from build123d import *

# Parameters (mm, degrees)
ESQUISSE1_W        = 256
ESQUISSE1_H        = 350
BOSS_EXTRU_1_DEPTH = 10
ESQUISSE2_W        = 256
ESQUISSE2_H        = 350
ESQUISSE2_W_2      = 236
ESQUISSE2_H_2      = 330
BOSS_EXTRU_2_DEPTH = 70
ESQUISSE3_W        = 10
ESQUISSE3_H        = 330
BOSS_EXTRU_3_DEPTH = 70


with BuildPart() as part:
    # Esquisse1 → Boss.-Extru.1 (new body)
    with BuildSketch(Plane.XY):
        with Locations((128, 175)):
            Rectangle(ESQUISSE1_W, ESQUISSE1_H)
    extrude(amount=BOSS_EXTRU_1_DEPTH)

    # Esquisse2 → Boss.-Extru.2 (add)
    with BuildSketch(Plane.XY.offset(10)):
        with Locations((128, 175)):
            Rectangle(ESQUISSE2_W, ESQUISSE2_H)
        with Locations((128, 175)):
            Rectangle(ESQUISSE2_W_2, ESQUISSE2_H_2, mode=Mode.SUBTRACT)
    extrude(amount=BOSS_EXTRU_2_DEPTH)

    # Esquisse3 → Boss.-Extru.3 (add)
    with BuildSketch(Plane.XY.offset(10)):
        with Locations((87, 175)):
            Rectangle(ESQUISSE3_W, ESQUISSE3_H)
        with Locations((169, 175)):
            Rectangle(ESQUISSE3_W, ESQUISSE3_H)
    extrude(amount=BOSS_EXTRU_3_DEPTH)


solid = part.part
Work out the finished part from the listing and answer in its coordinate system (mm). A direction names the side the tool comes from. Give positions to 0.01 mm unless a question says otherwise; leave off trailing zeros. Loops run counter-clockwise (first coordinate to the right, second up) from the corner with the lowest first, then second, coordinate; pieces in that order, holes last. Notation, with made-up numbers: (-0.75, 84) -> (39.25, 84) arc R22 ccw to (39.25, 115) -> close; hole circle Ø2 at (25.25, 3.25). An arc over 180 degrees is marked (long way). Use a Markdown table: item, result. Add a question column.
1) For a pull along Y with two mould halves and no side action, classify faces 1 (the flat face through (45, 340, 45)), 2 (the flat face through (0, 173, 39)), 3 (the flat face through (126, 350, 39)) as +Y half, -Y half, draft (parallel to the pull), parting line (faces both ways), or undercut.
2) The part is cut by section A-A, the plane z = 72. Determine the outline of the cut face in (x, y).
3) This flat-tipped pin is pushed along its axis until it touches: P1, Ø1.5, axis at x = 139.5, y = 45.5, coming from the +Z side. Where does it stop, or does it pass through?
4) The part is cut by section C-C, the plane x = 39. Determine the outline of the cut face in (y, z), plus the area to 3 significant figures.
5) The part is cut by section B-B, the plane y = 281.5. Determine the outline of the cut face in (x, z).
6) Which of the six approach directions +Z, -Z, +X, -X, +Y, -Y give full straight-line access (tool end or side, diameter ignored) to faces 4 (the flat face through (126, 177, 0)), 5 (the flat face through (127, 10, 45))?
7) Consider line 1 along X through (y, z) = (319, 31); line 2 along Y through (x, z) = (144.5, 60.5); line 3 along Z through (x, y) = (26, 146). Determine where each line is inside the solid, lowest interval first.
Reported:
| question | item | result |
|---|---|---|
| 1 | face 1 | undercut |
| 1 | face 2 | draft |
| 1 | face 3 | +Y half |
| 2 | outline | (0, 0) -> (256, 0) -> (256, 350) -> (0, 350) -> close; hole (10, 10) -> (82, 10) -> (82, 340) -> (10, 340) -> close; hole (92, 10) -> (164, 10) -> (164, 340) -> (92, 340) -> close; hole (174, 10) -> (246, 10) -> (246, 340) -> (174, 340) -> close |
| 3 | P1 | stops at z = 10 |
| 4 | outline | (0, 0) -> (350, 0) -> (350, 80) -> (340, 80) -> (340, 10) -> (10, 10) -> (10, 80) -> (0, 80) -> close |
| 4 | area | 4,900 mm^2 |
| 5 | outline | (0, 0) -> (256, 0) -> (256, 80) -> (246, 80) -> (246, 10) -> (174, 10) -> (174, 80) -> (164, 80) -> (164, 10) -> (92, 10) -> (92, 80) -> (82, 80) -> (82, 10) -> (10, 10) -> (10, 80) -> (0, 80) -> close |
| 6 | face 4 | -Z, +X, -X, +Y, -Y |
| 6 | face 5 | +Z |
| 7 | line 1 | x = 0 to 10, 82 to 92, 164 to 174, 246 to 256 |
| 7 | line 2 | y = 0 to 10, 340 to 350 |
| 7 | line 3 | z = 0 to 10 |
